```python
from build123d import *

# Parameters (mm, degrees)
SKETCH1_W                 = 93.58
SKETCH1_H                 = 68.18
BASE_DEPTH                = 5
SKETCH2_W                 = 93.58
SKETCH2_H                 = 68.18
WALLS_DEPTH               = 12
SKETCH2_4_R               = 1.07
SCREW_HOLES_DEPTH         = 5
SKETCH4_W                 = 4.45
SKETCH4_H                 = 38.18
SKETCH4_W_2               = 1.1
SKETCH4_W_3               = 63.58
SKETCH4_H_2               = 4.45
SKETCH4_H_3               = 1.1
WALLS_CUT_DEPTH           = 12
SKETCH4_3_W               = 5
SKETCH4_3_H               = 1.1
SKETCH4_3_W_2             = 1.1
SKETCH4_3_H_2             = 5
SKETCH4_3_W_3             = 63.58
SKETCH4_3_H_3             = 38.18
ACRYLIC_CUT_DEPTH         = 14
FILLET2_R                 = 5
FILLET3_R                 = 3
SKETCH5_W                 = 34
SKETCH5_H                 = 34
ARM_ATTACH_BODY_CUT_DEPTH = 1.5
SKETCH6_R                 = 2
CUT_EXTRUDE1_DEPTH        = 61.335994232


with BuildPart() as part:
    # Sketch1 → Base (new body)
    with BuildSketch(Plane(origin=(0, 0, 0), x_dir=(1, 0, 0), z_dir=(0, 1, 0))):
        Rectangle(SKETCH1_W, SKETCH1_H)
    extrude(amount=BASE_DEPTH)

    # Sketch2 → Walls (add)
    with BuildSketch(Plane(origin=(0, 5, 0), x_dir=(1, 0, 0), z_dir=(0, 1, 0))):
        Rectangle(SKETCH2_W, SKETCH2_H)
        Polygon((36.79, -2), (36.79, -24.09), (2, -24.09), (-2, -24.09), (-36.79, -24.09), (-36.79, -2), (-36.79, 2), (-36.79, 24.09), (-2, 24.09), (2, 24.09), (36.79, 24.09), (36.79, 2), align=None, mode=Mode.SUBTRACT)
    extrude(amount=WALLS_DEPTH)

    # Sketch2<4> → Screw Holes (add)
    with BuildSketch(Plane(origin=(0, 5, 0), x_dir=(1, 0, 0), z_dir=(0, 1, 0))):
        with Locations(Location((-5.04, 5.04, 0), (0, 0, 270))):
            Circle(SKETCH2_4_R)
        with Locations(Location((-34.25, 5.04, 0), (0, 0, 270))):
            Circle(SKETCH2_4_R)
        with Locations(Location((-34.25, 21.55, 0), (0, 0, 270))):
            Circle(SKETCH2_4_R)
        with Locations(Location((5.04, 21.55, 0), (0, 0, 90))):
            Circle(SKETCH2_4_R)
        with Locations(Location((5.04, 5.04, 0), (0, 0, 90))):
            Circle(SKETCH2_4_R)
        with Locations(Location((34.25, 5.04, 0), (0, 0, 90))):
            Circle(SKETCH2_4_R)
        with Locations(Location((34.25, 21.55, 0), (0, 0, 90))):
            Circle(SKETCH2_4_R)
        with Locations(Location((34.25, -5.04, 0), (0, 0, 270))):
            Circle(SKETCH2_4_R)
        with Locations(Location((34.25, -21.55, 0), (0, 0, 270))):
            Circle(SKETCH2_4_R)
        with Locations(Location((5.04, -21.55, 0), (0, 0, 270))):
            Circle(SKETCH2_4_R)
        with Locations(Location((5.04, -5.04, 0), (0, 0, 270))):
            Circle(SKETCH2_4_R)
        with Locations(Location((-5.04, -5.04, 0), (0, 0, 90))):
            Circle(SKETCH2_4_R)
        with Locations(Location((-34.25, -5.04, 0), (0, 0, 90))):
            Circle(SKETCH2_4_R)
        with Locations(Location((-34.25, -21.55, 0), (0, 0, 90))):
            Circle(SKETCH2_4_R)
        with Locations(Location((-5.04, -21.55, 0), (0, 0, 90))):
            Circle(SKETCH2_4_R)
        with Locations(Location((-5.04, 21.55, 0), (0, 0, 90))):
            Circle(SKETCH2_4_R)
    extrude(amount=SCREW_HOLES_DEPTH)

    # Sketch4 → Walls Cut (cut)
    with BuildSketch(Plane(origin=(0, 17, 0), x_dir=(1, 0, 0), z_dir=(0, 1, 0))):
        with Locations((39.015, 0)):
            Rectangle(SKETCH4_W, SKETCH4_H)
        with Locations((44.565, 0)):
            Rectangle(SKETCH4_W, SKETCH4_H)
        with Locations((41.79, 0)):
            Rectangle(SKETCH4_W_2, SKETCH4_H)
        with Locations((0, -26.315)):
            Rectangle(SKETCH4_W_3, SKETCH4_H_2)
        with Locations((0, -31.865)):
            Rectangle(SKETCH4_W_3, SKETCH4_H_2)
        with Locations((0, -29.09)):
            Rectangle(SKETCH4_W_3, SKETCH4_H_3)
        with Locations((0, 26.315)):
            Rectangle(SKETCH4_W_3, SKETCH4_H_2)
        with Locations((0, 29.09)):
            Rectangle(SKETCH4_W_3, SKETCH4_H_3)
        with Locations((0, 31.865)):
            Rectangle(SKETCH4_W_3, SKETCH4_H_2)
        with Locations((-39.015, 0)):
            Rectangle(SKETCH4_W, SKETCH4_H)
        with Locations((-44.565, 0)):
            Rectangle(SKETCH4_W, SKETCH4_H)
        with Locations((-41.79, 0)):
            Rectangle(SKETCH4_W_2, SKETCH4_H)
    extrude(amount=-WALLS_CUT_DEPTH, mode=Mode.SUBTRACT)

    # Sketch4<3> → Acrylic Cut (cut)
    with BuildSketch(Plane(origin=(0, 17, 0), x_dir=(1, 0, 0), z_dir=(0, 1, 0))):
        with Locations((34.29, 29.09)):
            Rectangle(SKETCH4_3_W, SKETCH4_3_H)
        with Locations((-34.29, 29.09)):
            Rectangle(SKETCH4_3_W, SKETCH4_3_H)
        with Locations((-41.79, 21.59)):
            Rectangle(SKETCH4_3_W_2, SKETCH4_3_H_2)
        with Locations((-41.79, -21.59)):
            Rectangle(SKETCH4_3_W_2, SKETCH4_3_H_2)
        with Locations((-34.29, -29.09)):
            Rectangle(SKETCH4_3_W, SKETCH4_3_H)
        with Locations((41.79, -21.59)):
            Rectangle(SKETCH4_3_W_2, SKETCH4_3_H_2)
        with Locations((34.29, -29.09)):
            Rectangle(SKETCH4_3_W, SKETCH4_3_H)
        with Locations((41.79, 21.59)):
            Rectangle(SKETCH4_3_W_2, SKETCH4_3_H_2)
        with Locations((0, -29.09)):
            Rectangle(SKETCH4_3_W_3, SKETCH4_3_H)
        with Locations((-41.79, 0)):
            Rectangle(SKETCH4_3_W_2, SKETCH4_3_H_3)
        with Locations((0, 29.09)):
            Rectangle(SKETCH4_3_W_3, SKETCH4_3_H)
        with Locations((41.79, 0)):
            Rectangle(SKETCH4_3_W_2, SKETCH4_3_H_3)
    extrude(amount=-ACRYLIC_CUT_DEPTH, mode=Mode.SUBTRACT)

    # Fillet2
    fillet2_edges = [part.edges().sort_by_distance(p)[0] for p in [
        (-46.79, 8.5, 34.09),
        (46.79, 8.5, 34.09),
        (46.79, 8.5, -34.09),
        (-46.79, 8.5, -34.09),
    ]]
    fillet(fillet2_edges, radius=FILLET2_R)

    # Fillet3
    fillet3_edges = [part.edges().sort_by_distance(p)[0] for p in [
        (46.79, 11, -19.09),
        (46.79, 11, 19.09),
        (31.79, 11, 34.09),
        (-31.79, 11, 34.09),
        (-31.79, 11, -34.09),
        (31.79, 11, -34.09),
        (-46.79, 11, 19.09),
        (-46.79, 11, -19.09),
    ]]
    fillet(fillet3_edges, radius=FILLET3_R)

    # Sketch5 → Arm Attach Body Cut (cut)
    with BuildSketch(Plane.XZ):
        Rectangle(SKETCH5_W, SKETCH5_H)
    extrude(amount=-ARM_ATTACH_BODY_CUT_DEPTH, mode=Mode.SUBTRACT)

    # Sketch6 → Cut-Extrude1 (cut, through all)
    with BuildSketch(Plane(origin=(0, 17, 0), x_dir=(1, 0, 0), z_dir=(0, 1, 0))):
        with Locations(Location((-41.79, 29.09, 0), (0, 0, 270))):
            Circle(SKETCH6_R)
        with Locations(Location((41.79, 29.09, 0), (0, 0, 90))):
            Circle(SKETCH6_R)
        with Locations(Location((41.79, -29.09, 0), (0, 0, 270))):
            Circle(SKETCH6_R)
        with Locations(Location((-41.79, -29.09, 0), (0, 0, 90))):
            Circle(SKETCH6_R)
    extrude(amount=-CUT_EXTRUDE1_DEPTH, mode=Mode.SUBTRACT)


solid = part.part
```
Input: part model. Units: mm. Frame: model coordinates. A direction names the side the tool comes from. Round coordinates to 2 decimals unless told otherwise and drop trailing zeros. Loops run counter-clockwise (first coordinate to the right, second up) from the corner with the lowest first, then second, coordinate; pieces in that order, holes last. Notation, with made-up numbers: (-11, 53) -> (23, 53) arc R33 ccw to (23, 81) -> close; hole circle Ø8 at (-2.5, 46.5). An arc over 180 degrees is marked (long way). Write each question's results on one line, items separated by ' | '.
1. Section C-C (x = 1). Return loops of the section in (y, z), and give its area (4 significant figures).
Geometry results:
outline: (0, -34.09) -> (5, -34.09) -> (5, -29.64) -> (3, -29.64) -> (3, -28.54) -> (5, -28.54) -> (5, 28.54) -> (3, 28.54) -> (3, 29.64) -> (5, 29.64) -> (5, 34.09) -> (0, 34.09) -> (0, 17) -> (1.5, 17) -> (1.5, -17) -> (0, -17) -> close | area: 285.5 mm2
2. Section D-D (x = 25). Return loops of the section in (y, z).
Geometry results:
outline: (0, -34.09) -> (5, -34.09) -> (5, -29.64) -> (3, -29.64) -> (3, -28.54) -> (5, -28.54) -> (5, 28.54) -> (3, 28.54) -> (3, 29.64) -> (5, 29.64) -> (5, 34.09) -> (0, 34.09) -> close
3. Section B-B (z = -12.5). Return loops of the section in (x, y).
Geometry results:
outline: (-46.79, 0) -> (-17, 0) -> (-17, 1.5) -> (17, 1.5) -> (17, 0) -> (46.79, 0) -> (46.79, 5) -> (42.34, 5) -> (42.34, 3) -> (41.24, 3) -> (41.24, 5) -> (-41.24, 5) -> (-41.24, 3) -> (-42.34, 3) -> (-42.34, 5) -> (-46.79, 5) -> close
4. Ray query, line 1 (Z direction, x = 22.5, y = 4); line 2 (X direction, y = 7.75, z = -29.09); line 3 (X direction, y = 10.25, z = -22). Return the intervals inside material, ascending. Write a range as from..to.
Geometry results:
line 1: -34.09..-29.64, -28.54..28.54, 29.64..34.09 | line 2: -46.79..-43.79, -39.79..-36.79, 36.79..39.79, 43.79..46.79 | line 3: -46.79..-42.34, -41.24..-36.79, 36.79..41.24, 42.34..46.79
5. First-contact query: P1, Ø2, axis at x = -6, z = 9, coming from the +Y side; P2, Ø1.2, axis at y = 10, z = 30.5, coming from the +X side; P3, Ø1.5, axis at x = -34.5, y = 8, coming from the +Z side; P4, Ø7, axis at x = 8, y = 9, coming from the +Z side. Flat tips, straight axial feed; report the tip coordinate or a pass-through.
Geometry results:
P1: y = 5 | P2: x = 46.72 | P3: z = 34.09 | P4: z = 22.62
6. Section A-A (y = 12). State how many separate pieces and enclosed holes the cut face has, and give its area (3 significant figures).
Geometry results:
separate pieces: 4 | enclosed holes: 4 | area: 669 mm2
7. Set-up query: faces 1 (the face through (39, 11, -19.09)), 2 (the face through (-32.69, 10.92, 33.23)), 3 (the face through (34, 10, 22)), 4 (the face through (-39, 17, 26)), 5 (the face through (5, 10, 22)). Return all of +Z, -Z, +X, -X, +Y, -Y with unobstructed straight access to the full face (end or side cutting, diameter ignored); none if empty.
Geometry results:
face 1: +X, -X, +Y | face 2: +Z, +Y | face 3: +Y | face 4: +Z, -Z, +X, -X, +Y | face 5: +Z, -Z, +Y
8. Mould query, pull axis X, two halves, no side actions, for faces 6 (the face through (-21, 0, 0)), 7 (the face through (45.93, 10.92, -19.99)), 8 (the face through (0, 4, -29.64)), 9 (the face through (-45.36, 8.62, 32.59)). Classes: +X half, -X half, draft (parallel to the pull), parting line (faces both ways), or undercut.
Geometry results:
face 6: draft | face 7: +X half | face 8: undercut | face 9: -X half
